For this review, take the finished solid that the model builds, in its own axes (mm). Give positions to 0.01 mm unless a question says otherwise; leave off trailing zeros. Loops run counter-clockwise (first coordinate to the right, second up) from the corner with the lowest first, then second, coordinate; pieces in that order, holes last. Notation, with made-up numbers: (23, 46.5) - (42, 46.5) arc R12 ccw to (42, 64.5) - close; hole circle Ø5 at (84.5, 77.25). An arc over 180 degrees is marked (long way). Answer in a Markdown table with one row per item.
```python
from build123d import *

# Parameters (mm, degrees)
BASE_FLANGE1_DEPTH = 2.65684


# Sheet-metal steps are written as plain solids
with BuildPart() as part:
    # Sketch1 → Base-Flange1 (new body)
    with BuildSketch(Plane.XY):
        with BuildLine():
            Line((-177.8, 0), (-12.7, 0))
            ThreePointArc((-12.7, 0), (0, 12.7), (12.7, 0))
            Line((12.7, 0), (177.8, 0))
            ThreePointArc((177.8, 0), (125.723585695, 125.723585695), (0, 177.8))
            ThreePointArc((0, 177.8), (-125.723585695, 125.723585695), (-177.8, 0))
        make_face()
    extrude(amount=-BASE_FLANGE1_DEPTH)


solid = part.part
```
1. Wall thickness on line 1 (Y direction, x = 136.5, z = -0.2); line 2 (Y direction, x = 42, z = -2.5); line 3 (X direction, y = 52.5, z = -2.3): over which ranges is each line inside the solid? List them lowest first. Write a range as [from, to].
Values:
| item | result |
|---|---|
| line 1 | y = [0, 113.93] |
| line 2 | y = [0, 172.77] |
| line 3 | x = [-169.87, 169.87] |
2. We need section B-B, the plane x = 155.5. Give the boundary of the cut face in (y, z).
Values:
| item | result |
|---|---|
| outline | (0, -2.66) - (86.21, -2.66) - (86.21, 0) - (0, 0) - close |
3. Mouldability with a two-part tool opening along X and no side actions: class faces 1 (the face through (-0.279, 12.697, -1.31)), 2 (the face through (-2, 70, 0)) as released by +X, released by -X, zero draft, split by the parting line, or undercut.
Values:
| item | result |
|---|---|
| face 1 | undercut |
| face 2 | zero draft |
4. Clearance check with flat-ended pins moving along their axes: pin 1 (1.5 mm diameter, centred on y = 36, z = -0.5, fed in from +X); pin 2 (1.5 mm diameter, centred on y = 128.5, z = -1, fed in from +X); pin 3 (1 mm diameter, centred on y = 144.5, z = -1.5, fed in from +X). State where each tip first meets the part, or that it passes through.
Values:
| item | result |
|---|---|
| pin 1 | stops at x = 174.27 |
| pin 2 | stops at x = 123.66 |
| pin 3 | stops at x = 104.29 |
5. We need section C-C, the plane y = 148. Give the boundary of the cut face in (x, z).
Values:
| item | result |
|---|---|
| outline | (-98.53, -2.66) - (98.53, -2.66) - (98.53, 0) - (-98.53, 0) - close |
6. We need section A-A, the plane z = -1.8. Give the boundary of the cut face in (x, y).
Values:
| item | result |
|---|---|
| outline | (-177.8, 0) - (-12.7, 0) arc R12.7 cw to (12.7, 0) - (177.8, 0) arc R177.8 ccw to start |
